Could you check a few things on this model? Use its own coordinates, in mm. Face numbers are marked on the shaded views. Coordinates: 2 decimals unless noted, no trailing zeros. Order: outer loops, then holes, each group sorted by start corner. A loop starts at its lowest first (then second) coordinate and runs counter-clockwise, first axis right, second up. Notation, with made-up numbers: (-37, 44) - (-15, 44) arc R25 ccw to (-15, 70) - close; hole circle Ø1 at (40, 86). An arc over 180 degrees is marked (long way). One line per item, written item: value.
from build123d import *

# Parameters (mm, degrees)
SKETCH_1_R          = 6
SKETCH_1_R_2        = 3
EXTRUDE_1_DEPTH     = 10
SKETCH_2_W          = 10
SKETCH_2_H          = 12
SKETCH_2_R          = 3.5
EXTRUDE_2_DEPTH     = 13
CUT_EXTRUDE_START   = -13
SKETCH_4_R          = 3
CUT_EXTRUDE_1_DEPTH = 13
CUT_EXTRUDE_START_2 = -8.5
SKETCH_5_R          = 3.5
CUT_EXTRUDE_2_DEPTH = 8.5


with BuildPart() as part:
    # 草图1 → 凸台-拉伸1 (new body)
    with BuildSketch(Plane(origin=(0, 0, 0), x_dir=(0, 0, -1), z_dir=(1, 0, 0))):
        Circle(SKETCH_1_R)
        Circle(SKETCH_1_R_2, mode=Mode.SUBTRACT)
    extrude(amount=EXTRUDE_1_DEPTH)

    # 草图2 → 凸台-拉伸2 (add)
    with BuildSketch(Plane(origin=(0, 0, 0), x_dir=(1, 0, 0), z_dir=(0, 1, 0))):
        with Locations((5, 0)):
            Rectangle(SKETCH_2_W, SKETCH_2_H)
        with Locations(Location((5, 0, 0), (0, 0, 90))):
            Circle(SKETCH_2_R, mode=Mode.SUBTRACT)
    extrude(amount=EXTRUDE_2_DEPTH)

    # 草图4 → 切除-拉伸1 (cut)
    with BuildSketch(Plane(origin=(10, 0, 0), x_dir=(0, 0, -1), z_dir=(1, 0, 0)).offset(CUT_EXTRUDE_START)):
        Circle(SKETCH_4_R)
    extrude(amount=CUT_EXTRUDE_1_DEPTH, mode=Mode.SUBTRACT)

    # 草图5 → 切除-拉伸2 (cut)
    with BuildSketch(Plane(origin=(0, 13, 0), x_dir=(1, 0, 0), z_dir=(0, 1, 0)).offset(CUT_EXTRUDE_START_2)):
        with Locations(Location((5, 0, 0), (0, 0, 90))):
            Circle(SKETCH_5_R)
    extrude(amount=CUT_EXTRUDE_2_DEPTH, mode=Mode.SUBTRACT)


solid = part.part
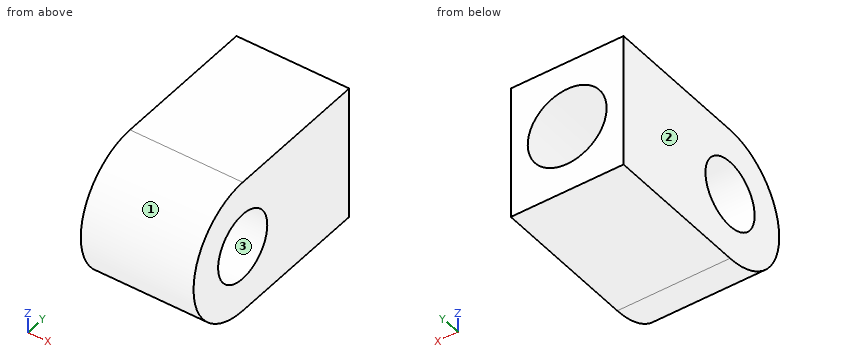
Item 1: Thinking about a two-plate mould opening in Y: for the marked faces 1, 2 and 3, which applies, pulls with the +Y half, pulls with the -Y half, needs draft (parallel to the pull), parting line crosses it, or undercut?
Conclusion:
face 1: pulls with the -Y half
face 2: needs draft
face 3: undercut
Item 2: I want a section at C-C on y = 8. Please give me the cut outline in (x, z).
Conclusion:
outline: (0, -6) - (10, -6) - (10, 6) - (0, 6) - close; hole circle Ø7 at (5, 0)
Item 3: I'm going to push flat-ended pins straight in: pin 1 Ø1 at (x, z) = (1.5, 2.5) entering from -Y; pin 2 Ø2 at (x, z) = (5.5, 1) entering from +Y. Where does each tip first touch, or does it pass through?
Conclusion:
pin 1: y = -5.66
pin 2: y = 4.5
Item 4: I want a section at D-D on y = -0.5. Please give me the cut outline in (x, z).
Conclusion:
outline: (0, -5.98) - (10, -5.98) - (10, -2.96) - (0, -2.96) - close; (0, 2.96) - (10, 2.96) - (10, 5.98) - (0, 5.98) - close
Item 5: I want a section at B-B on x = 5. Please give me the cut outline in (y, z), then the cut area to 3 significant figures.
Conclusion:
outline: (0, -6) - (13, -6) - (13, -3.5) - (4.5, -3.5) - (4.5, 3.5) - (13, 3.5) - (13, 6) - (0, 6) arc R6 ccw to start; hole circle Ø6 at (0, 0)
area: 125 mm²
Item 6: I want a section at A-A on z = 0. Please give me the cut outline in (x, y).
Conclusion:
outline: (0, -6) - (10, -6) - (10, -3) - (0, -3) - close; (0, 3) - (10, 3) - (10, 13) - (8.5, 13) - (8.5, 4.5) - (1.5, 4.5) - (1.5, 13) - (0, 13) - close
Item 7: If I drill on probe 1 along X at (y, z) = (5.15, 0); probe 2 along Y at (x, z) = (4, 0); probe 3 along Z at (x, y) = (8, 7.75), over which ranges is the centre line in solid material (lowest first)?
Conclusion:
probe 1: 0 to 1.5, 8.5 to 10
probe 2: -6 to -3, 3 to 4.5
probe 3: -6 to -1.8, 1.8 to 6
